```python
from build123d import *


with BuildPart() as part:
    # Sketch1 → Revolve1 (revolve)
    with BuildSketch(Plane(origin=(0, 0, 0), x_dir=(1, 0, 0), z_dir=(0, 1, 0))):
        with BuildLine():
            Line((0, 12.7), (0, 10.795))
            ThreePointArc((0, 10.795), (7.633217703, 7.633217703), (10.795, 0))
            Line((10.795, 0), (12.7, 0))
            ThreePointArc((12.7, 0), (12.597580707, 1.609646024), (12.291974752, 3.193330031))
            Line((12.291974752, 3.193330031), (136.525, 3.193330031))
            Line((136.525, 3.193330031), (136.525, 7.62))
            Line((136.525, 7.62), (10.16, 7.62))
            ThreePointArc((10.16, 7.62), (5.679612663, 11.359225326), (0, 12.7))
        make_face()
    revolve(axis=Axis((0, 0, 0), (1, 0, 0)))


solid = part.part
```
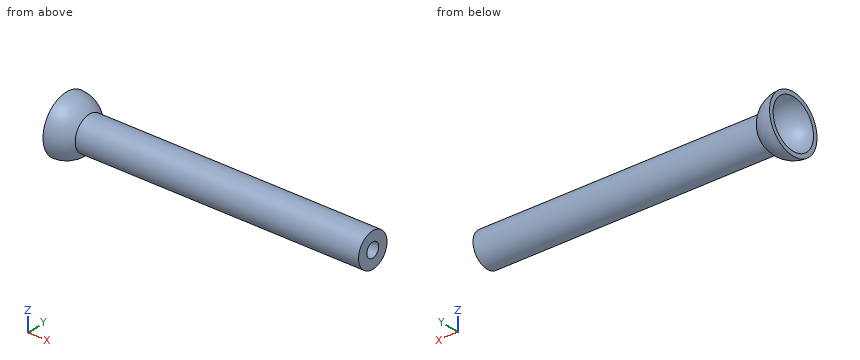
Geometry check sheet. Reference: the model listing, model coordinates, mm. Round coordinates to 2 decimals unless told otherwise and drop trailing zeros. Write each loop counter-clockwise with the first axis right and the second up, starting at its lowest first coordinate (ties: lowest second). Pieces come first, ordered by that corner, then holes. Notation, with made-up numbers: (83.5, 47.5) -> (122.5, 47.5) arc R6 ccw to (122.5, 54.5) -> close; hole circle Ø10 at (2.25, 73). An arc over 180 degrees is marked (long way). Put each result on its own line as item: value.
1) Cross-section at C-C, the plane x = 96. Enter the section's corners in (y, z).
Recorded:
outline: circle Ø15.24 at (0, 0); hole circle Ø6.39 at (0, 0)
2) Depth check by flat-ended pin: P1, Ø1.5, axis at x = 95, y = 0, coming from the +Z side; P2, Ø12, axis at x = 24, y = 9.5, coming from the +Z side; P3, Ø5, axis at y = 0, z = 0, coming from the -X side. Enter the tip coordinate at first touch or a pass-through.
Recorded:
P1: stops at z = 7.62
P2: stops at z = 6.77
P3: stops at x = 10.5
3) Cross-section at D-D, the plane z = 5.5. Enter the section's corners in (x, y) (3 decimals).
Recorded:
outline: (0, -11.447) arc R11.447 ccw to (10.16, -5.274) -> (136.525, -5.274) -> (136.525, 5.274) -> (10.16, 5.274) arc R11.447 ccw to (0, 11.447) -> (0, 9.289) arc R9.289 cw to (0, -9.289) -> close
4) Thickness scan on probe 1 along Y at (x, z) = (85, 0); probe 2 along Z at (x, y) = (119.5, -2.75). Record the ranges inside material, lowest first. Write a range as from..to.
Recorded:
probe 1: y = -7.62..-3.19, 3.19..7.62
probe 2: z = -7.11..-1.62, 1.62..7.11
5) Cross-section at A-A, the plane y = 0. Enter the section's corners in (x, z) (3 decimals), plus the area to 3 significant figures.
Recorded:
outline: (0, -12.7) arc R12.7 ccw to (10.16, -7.62) -> (136.525, -7.62) -> (136.525, -3.193) -> (12.292, -3.193) arc R12.7 ccw to (12.292, 3.193) -> (136.525, 3.193) -> (136.525, 7.62) -> (10.16, 7.62) arc R12.7 ccw to (0, 12.7) -> (0, 10.795) arc R10.795 cw to (0, -10.795) -> close
area: 1,180 mm2
